```python
from build123d import *

# Parameters (mm, degrees)
BOSS_EXTRUDE1_DEPTH = 5
SKETCH5_W           = 4
SKETCH5_H           = 15
BOSS_EXTRUDE2_DEPTH = 13.5
SKETCH6_W           = 4
SKETCH6_H           = 15
BOSS_EXTRUDE3_DEPTH = 7.5
SKETCH7_W           = 56.316926488
SKETCH7_H           = 4.75
BOSS_EXTRUDE4_DEPTH = 5.2
SKETCH8_W           = 56.316926488
SKETCH8_H           = 9.75
BOSS_EXTRUDE5_DEPTH = 4.5


with BuildPart() as part:
    # Sketch4 → Boss-Extrude1 (new body)
    with BuildSketch(Plane(origin=(0, 0, 0), x_dir=(0, 0, -1), z_dir=(1, 0, 0))):
        Polygon((-207.602722557, -7.920601616), (-252.602722557, -7.920601616), (-252.602722557, -22.920601616), (-148.102722557, -22.920601616), (-148.102722557, 28.079398384), (-252.602722557, 28.079398384), (-252.602722557, 13.079398384), (-207.602722557, 13.079398384), align=None)
    extrude(amount=BOSS_EXTRUDE1_DEPTH)

    # Sketch5 → Boss-Extrude2 (add)
    with BuildSketch(Plane(origin=(5, 0, 0), x_dir=(0, 0, -1), z_dir=(1, 0, 0))):
        with Locations((-250.602722557, 20.579398384)):
            Rectangle(SKETCH5_W, SKETCH5_H)
        with Locations((-250.602722557, -15.420601616)):
            Rectangle(SKETCH5_W, SKETCH5_H)
    extrude(amount=BOSS_EXTRUDE2_DEPTH)

    # Sketch6 → Boss-Extrude3 (add)
    with BuildSketch(Plane(origin=(0, 0, 248.602722557), x_dir=(-1, 0, 0), z_dir=(0, 0, -1))):
        with Locations((-16.5, -15.420601616)):
            Rectangle(SKETCH6_W, SKETCH6_H)
        with Locations((-16.5, 20.579398384)):
            Rectangle(SKETCH6_W, SKETCH6_H)
    extrude(amount=BOSS_EXTRUDE3_DEPTH)

    # Sketch7 → Boss-Extrude4 (add)
    with BuildSketch(Plane.ZY):
        with Locations((176.261185801, 17.829398384)):
            Rectangle(SKETCH7_W, SKETCH7_H)
    boss_extrude4 = extrude(amount=BOSS_EXTRUDE4_DEPTH)

    # Sketch8 → Boss-Extrude5 (add)
    with BuildSketch(Plane.ZY.offset(5.2)):
        with Locations((176.261185801, 17.829398384)):
            Rectangle(SKETCH8_W, SKETCH8_H)
    boss_extrude5 = extrude(amount=BOSS_EXTRUDE5_DEPTH)

    # Mirror1: Boss-Extrude4, Boss-Extrude5 across plane
    add(boss_extrude4.mirror(Plane(origin=(0, 2.579398384, 0), x_dir=(0, 0, 1), z_dir=(0, -1, 0))))
    add(boss_extrude5.mirror(Plane(origin=(0, 2.579398384, 0), x_dir=(0, 0, 1), z_dir=(0, -1, 0))))


solid = part.part
```
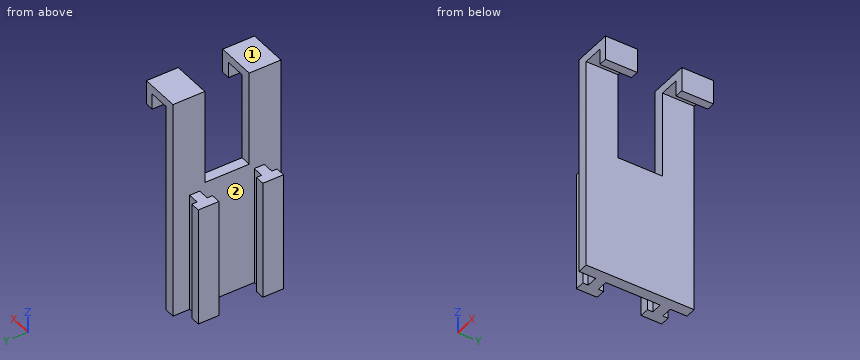
The model under review builds one solid part; all positions refer to its coordinate system, in mm. Face numbers are marked on the shaded views. A direction names the side the tool comes from. Coordinates: 2 decimals unless noted, no trailing zeros. Write each loop counter-clockwise with the first axis right and the second up, starting at its lowest first coordinate (ties: lowest second). Pieces come first, ordered by that corner, then holes.
1) Machinability: for the marked faces 1 and 2, which of the approach directions +Z, -Z, +X, -X, +Y, -Y give a long, thin tool a straight path to every point of the face, cutting with its end or side? Answer none if there is none.
2) We need section B-B on x = -7.25. State the section outline as (y, z) points, then the cut area to 3 significant figures.
3) We need section A-A on z = 239.5. State the section outline as (x, y) points.
4) We need section C-C on y = 17. State the section outline as (x, z) points, then the cut area to 3 significant figures.
5) We need section D-D on x = 3. State the section outline as (y, z) points.
6) Clearance check with flat-ended pins moving along their axes: pin 1 Ø8 at (y, z) = (24, 244) entering from -X; pin 2 Ø2 at (y, z) = (21.5, 179.5) entering from +X; pin 3 Ø1.2 at (x, y) = (16, 20) entering from -Z. State where each tip first meets the part, or that it passes through.
7) To check wall thickness, follow probe 1 along Y at (x, z) = (4, 214.5); probe 2 along X at (y, z) = (-19.5, 236); probe 3 along X at (y, z) = (20, 245). State the ranges of each line that lie inside material, in increasing order.
Answer list:
1. face 1: +Z, +X, -X, +Y, -Y
1. face 2: +Z
2. outline: (-17.55, 148.1) - (-7.8, 148.1) - (-7.8, 204.42) - (-17.55, 204.42) - close; (12.95, 148.1) - (22.7, 148.1) - (22.7, 204.42) - (12.95, 204.42) - close
2. area: 1,100 mm2
3. outline: (0, -22.92) - (5, -22.92) - (5, -7.92) - (0, -7.92) - close; (0, 13.08) - (5, 13.08) - (5, 28.08) - (0, 28.08) - close
4. outline: (-9.7, 148.1) - (5, 148.1) - (5, 248.6) - (14.5, 248.6) - (14.5, 241.1) - (18.5, 241.1) - (18.5, 252.6) - (0, 252.6) - (0, 204.42) - (-9.7, 204.42) - close
4. area: 1,150 mm2
5. outline: (-22.92, 148.1) - (28.08, 148.1) - (28.08, 252.6) - (13.08, 252.6) - (13.08, 207.6) - (-7.92, 207.6) - (-7.92, 252.6) - (-22.92, 252.6) - close
6. pin 1: stops at x = 0
6. pin 2: stops at x = 5
6. pin 3: stops at z = 241.1
7. probe 1: y = -22.92 to -7.92, 13.08 to 28.08
7. probe 2: x = 0 to 5
7. probe 3: x = 0 to 5, 14.5 to 18.5
